Input: part model. Units: mm. Frame: model coordinates. A direction names the side the tool comes from. Round coordinates to 2 decimals unless told otherwise and drop trailing zeros. Order: outer loops, then holes, each group sorted by start corner. A loop starts at its lowest first (then second) coordinate and runs counter-clockwise, first axis right, second up. Notation, with made-up numbers: M 41.25,72.25 L 96.25,72.25 A23 cw 96.25,82.25 Z; hole C 74,38 d9. An arc over 180 degrees is marked long. One line per question, with ' | ' between items.
```python
from build123d import *

# Parameters (mm, degrees)
F0_W     = 213.626973
F0_H     = 116.731882
F1_DEPTH = 25.4
F2_W     = 33.02
F2_H     = 33.02
F3_DEPTH = 121.666
F5_D     = 25.4


with BuildPart() as f1:
    # F0 (on Front) → F1 (new body)
    with BuildSketch(Plane.XZ):
        with Locations((-9.536925, -10.872088)):
            Rectangle(F0_W, F0_H)
    extrude(amount=F1_DEPTH)

    # F2 (on face) → F3 (join)
    with BuildSketch(Plane.XZ.offset(25.4)):
        with Locations((-99.840412, 30.983853)):
            Rectangle(F2_W, F2_H)
        with Locations((80.766561, 30.983853)):
            Rectangle(F2_W, F2_H)
        with Locations((80.766561, -52.728029)):
            Rectangle(F2_W, F2_H)
        with Locations((-99.840412, -52.728029)):
            Rectangle(F2_W, F2_H)
    extrude(amount=F3_DEPTH)

    # F5 (through all)
    with Locations(Plane(origin=(0, 0, 0), x_dir=(-1, 0, 0), z_dir=(0, 1, 0))):
        with Locations((0, 0)):
            Hole(F5_D / 2)


solid = f1.part
```
Item 1: Section query A-A, the plane y = -38. Return loops of the section in (x, z).
Report:
outline: M -116.35,-69.24 L -83.33,-69.24 L -83.33,-36.22 L -116.35,-36.22 Z; M -116.35,14.47 L -83.33,14.47 L -83.33,47.49 L -116.35,47.49 Z; M 64.26,-69.24 L 97.28,-69.24 L 97.28,-36.22 L 64.26,-36.22 Z; M 64.26,14.47 L 97.28,14.47 L 97.28,47.49 L 64.26,47.49 Z
Item 2: Section query D-D, the plane x = 77. Return loops of the section in (y, z).
Report:
outline: M -147.07,-69.24 L 0,-69.24 L 0,47.49 L -147.07,47.49 L -147.07,14.47 L -25.4,14.47 L -25.4,-36.22 L -147.07,-36.22 Z
Item 3: Section query B-B, the plane x = 0. Return loops of the section in (y, z), plus the area to 3 significant figures.
Report:
outline: M -25.4,-69.24 L 0,-69.24 L 0,-12.7 L -25.4,-12.7 Z; M -25.4,12.7 L 0,12.7 L 0,47.49 L -25.4,47.49 Z | area: 2,320 mm²
Item 4: Access query for faces 1 (the flat face through (97.277, -85, -53)), 2 (the flat face through (-100, -85, -36.218)), 3 (the flat face through (-83.33, -85, -53)). Directions: +Z, -Z, +X, -X, +Y, -Y. A direction counts if a zero-diameter tool reaches every point of the face in a straight line with its end or side. Return the directions, or none.
Report:
face 1: +Z, -Z, +X, +Y, -Y | face 2: +X, -X, -Y | face 3: +Z, -Z, -Y
Item 5: Mould query, pull axis Z, two halves, no side actions, for faces 4 (the cylindrical face through (-2.75, -12.88, -12.4)), 5 (the flat face through (-11, -23, 47.494)), 6 (the flat face through (-100, -85, 14.474)), 7 (the flat face through (-100, -147.066, -52)). Classes: +Z half, -Z half, draft (parallel to the pull), parting line (faces both ways), or undercut.
Report:
face 4: undercut | face 5: +Z half | face 6: undercut | face 7: draft
Item 6: Section query C-C, the plane z = 0. Return loops of the section in (x, y).
Report:
outline: M -116.35,-25.4 L -12.7,-25.4 L -12.7,0 L -116.35,0 Z; M 12.7,-25.4 L 97.28,-25.4 L 97.28,0 L 12.7,0 Z
Item 7: First-contact query: pin 1 (2 mm diameter, centred on x = -81.5, z = 1.5, fed in from -Y). Flat tip, straight axial feed; report the tip coordinate or a pass-through.
Report:
pin 1: y = -25.4
Item 8: Line query: line 1 along Z through (x, y) = (84, -73); line 2 along X through (y, z) = (-113.5, -46.5); line 3 along Z through (x, y) = (0, -14.25). Output: solid intervals per line, ascending. Write a range as from..to.
Report:
line 1: -69.24..-36.22, 14.47..47.49 | line 2: -116.35..-83.33, 64.26..97.28 | line 3: -69.24..-12.7, 12.7..47.49
